The model under review builds one solid part; all positions refer to its coordinate system, in mm. Face numbers are marked on the shaded views. A direction names the side the tool comes from. Round coordinates to 2 decimals unless told otherwise and drop trailing zeros. Write each loop counter-clockwise with the first axis right and the second up, starting at its lowest first coordinate (ties: lowest second). Pieces come first, ordered by that corner, then holes. Notation, with made-up numbers: (69.5, 47) - (106.5, 47) arc R28 cw to (106.5, 72) - close; hole circle Ø7 at (89.25, 62.5). An arc over 180 degrees is marked (long way). Return JSON: item names as keys, results as strings.
from build123d import *

# Parameters (mm, degrees)
CYLINDER003_R     = 3
CYLINDER003_DEPTH = 10
PAD008_DEPTH      = 10
SKETCH032_R       = 1.625
POCKET023_DEPTH   = 55.910244
SKETCH033_W       = 20
SKETCH033_H       = 7
PAD009_DEPTH      = 7.5
SKETCH034_R       = 1.375
POCKET024_DEPTH   = 12
CHAMFER020_1_SIZE = 3.5
CHAMFER020_2_SIZE = 1
CHAMFER021_SIZE   = 0.5
CHAMFER022_SIZE   = 2


with BuildPart() as boardbracketscrewheadcylinder:
    # Cylinder003 → Cylinder003 (new body)
    with BuildSketch(Plane(origin=(0, 0.5, 24), x_dir=(1, 0, 0), z_dir=(0, 0, 1))):
        Circle(CYLINDER003_R)
    extrude(amount=CYLINDER003_DEPTH)


with BuildPart() as boardbracketpinschamfer022_final:
    # Sketch031 → Pad008 (new body, symmetric)
    with BuildSketch(Plane.YZ):
        Polygon((4.5, 21), (4.5, 24.911688), (-4.23971, 33.651398), (-7.975533, 34.909244), (-9.918525, 32.966252), (-9.211418, 32.259145), (-8.150758, 33.319805), (-5.32233, 31.905592), (-1.07969, 27.662951), (-25.828427, 2.914214), (-30.071068, 7.156854), (-31.485281, 9.985281), (-30.424621, 11.045942), (-31.131728, 11.753048), (-33.07472, 9.810056), (-31.714777, 5.972136), (-4.742641, -21), (4.5, -21), (4.5, -18), (-3.5, -18), (-23, 1.5), (-3.5, 21), align=None)
    extrude(amount=PAD008_DEPTH, both=True)

    # Sketch032 → Pocket023 (cut, through all)
    with BuildSketch(Plane.YX.offset(21)):
        with Locations((0.5, 0)):
            Circle(SKETCH032_R)
    extrude(amount=-POCKET023_DEPTH, mode=Mode.SUBTRACT)

    # Cut001: cut BoardBracketScrewHeadCylinder
    add(boardbracketscrewheadcylinder.part, mode=Mode.SUBTRACT)

    # Sketch033 → Pad009 (new body)
    with BuildSketch(Plane(origin=(0, -12.87132, -12.87132), x_dir=(1, 0, 0), z_dir=(0, -0.707107, -0.707107))):
        with Locations((0, 22.75)):
            Rectangle(SKETCH033_W, SKETCH033_H)
        with Locations((0, -7.5)):
            Rectangle(SKETCH033_W, SKETCH033_H)
    extrude(amount=PAD009_DEPTH)

    # Sketch034 → Pocket024 (cut)
    with BuildSketch(Plane(origin=(0, -18.174621, -18.174621), x_dir=(1, 0, 0), z_dir=(0, -0.707107, -0.707107))):
        with Locations((3.25, 22.75)):
            Circle(SKETCH034_R)
    pocket024 = extrude(amount=-POCKET024_DEPTH, mode=Mode.SUBTRACT)

    # Mirrored002: Pocket024 across Sketch034 V_Axis
    add(pocket024.mirror(Plane(origin=(0, -18.174621, -18.174621), x_dir=(0, -0.707107, -0.707107), z_dir=(1, 0, 0))), mode=Mode.SUBTRACT)

    # Chamfer020 1
    chamfer020_1_edges = [boardbracketpinschamfer022_final.edges().sort_by_distance(p)[0] for p in [
        (-10, -12.87132, -23.477922),
        (10, -12.87132, -23.477922),
    ]]
    chamfer(chamfer020_1_edges, length=CHAMFER020_1_SIZE)

    # Chamfer020 2
    chamfer020_2_edges = [boardbracketpinschamfer022_final.edges().sort_by_distance(p)[0] for p in [
        (-1.875, -34.2613, -2.087942),
        (1.875, -34.2613, -2.087942),
    ]]
    chamfer(chamfer020_2_edges, length=CHAMFER020_2_SIZE)

    # Chamfer021
    chamfer021_edges = [boardbracketpinschamfer022_final.edges().sort_by_distance(p)[0] for p in [
        (10, -4.917893, -20.824747),
        (10, -0.12132, -21),
        (10, 4.5, -19.5),
        (10, 0.5, -18),
        (10, -13.25, -8.25),
        (10, -13.25, 11.25),
        (10, 0.5, 21),
        (10, 4.5, 22.955844),
        (10, -30.778175, 8.571068),
        (10, -27.949747, 5.035534),
        (10, -13.454058, 15.288582),
        (10, -3.20101, 29.784271),
        (10, -6.736544, 32.612698),
    ]]
    chamfer(chamfer021_edges, length=CHAMFER021_SIZE)

    # Chamfer022
    chamfer022_edges = [boardbracketpinschamfer022_final.edges().sort_by_distance(p)[0] for p in [
        (8.25, -14.108757, -19.765611),
        (-8.25, -14.108757, -19.765611),
    ]]
    chamfer(chamfer022_edges, length=CHAMFER022_SIZE)


solid = boardbracketpinschamfer022_final.part
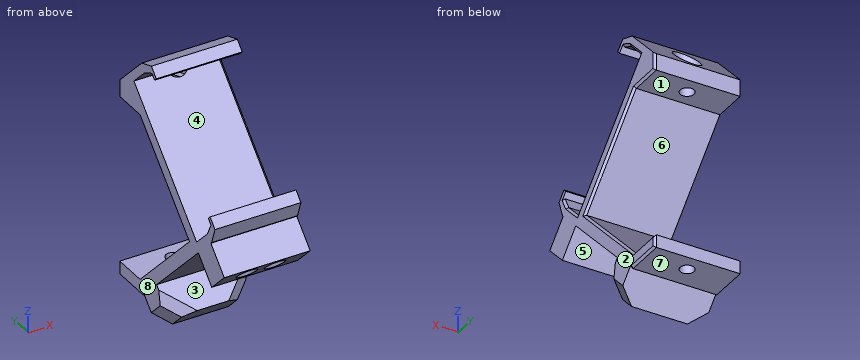
(1) Add section D-D (x = 0). Give the number of separate pieces and of enclosed holes in the cut face, plus the area to 3 significant figures.
Filled in:
{"separate pieces": "4", "enclosed holes": "0", "area": "355 mm2"}
(2) For the marked faces 1, 2, 3, 4 and 5, list the 3-axis set-ups (+Z, -Z, +X, -X, +Y, -Y) from which the entire face can be reached by the end or side of a thin tool; tool diameter is ignored.
Filled in:
{"face 1": "+X, -X, +Y", "face 2": "+Z, -Z, +X, +Y, -Y", "face 3": "+X, -X, -Y", "face 4": "+X, -X", "face 5": "-Z, +X, -X"}
(3) Add section A-A (y = -18). Write out the cut boundary in (x, z).
Filled in:
{"outline": "(-10, -7.74) - (10, -7.74) - (10, -4.21) - (9.5, -3.5) - (-10, -3.5) - close; (-10, 6.5) - (9.5, 6.5) - (10, 7.21) - (10, 10.04) - (9.5, 10.74) - (-10, 10.74) - close"}
(4) Clearance check with flat-ended pins moving along their axes: pin 1 Ø1.5 at (x, z) = (7, -15) entering from +Y; pin 2 Ø4 at (x, y) = (0, 0.5) entering from +Z; pin 3 Ø8 at (x, y) = (0, 0.5) entering from -Z. State where each tip first meets the part, or that it passes through.
Filled in:
{"pin 1": "stops at y = -5.75", "pin 2": "stops at z = 24", "pin 3": "stops at z = -21"}
(5) Mouldability with a two-part tool opening along Z and no side actions: class the marked faces 6, 7 and 8 as released by +Z, released by -Z, zero draft, split by the parting line, or undercut.
Filled in:
{"face 6": "undercut", "face 7": "released by -Z", "face 8": "zero draft"}
(6) Add section C-C (z = 19). Write out the cut boundary in (x, y), plus the area to 3 significant figures.
Filled in:
{"outline": "(-10, -9.74) - (9.5, -9.74) - (10, -9.04) - (10, -6.21) - (9.5, -5.5) - (-10, -5.5) - close", "area": "84.5 mm2"}
(7) Wall thickness on line 1 (Z direction, x = 8.75, y = -10.5); line 2 (Z direction, x = 9, y = -9); line 3 (X direction, y = 0, z = 22): over which ranges is each line inside the solid? List them lowest first.
Filled in:
{"line 1": "z = -22.67 to -16.16, -15.24 to -11, 14 to 18.24", "line 2": "z = -23.81 to -12.5, 15.5 to 19.74, 32.47 to 33.88", "line 3": "x = -10 to -1.55, 1.55 to 10"}
(8) Add section B-B (y = 0.5). Write out the cut boundary in (x, z) (3 decimals), plus the area to 3 significant figures.
Filled in:
{"outline": "(-10, -21) - (-1.625, -21) - (-1.625, -18) - (-10, -18) - close; (-10, 21) - (-1.625, 21) - (-1.625, 24) - (-3, 24) - (-3, 28.912) - (-10, 28.912) - close; (1.625, -21) - (9.5, -21) - (10, -20.5) - (10, -18.5) - (9.5, -18) - (1.625, -18) - close; (1.625, 21) - (9.5, 21) - (10, 21.5) - (10, 28.912) - (3, 28.912) - (3, 24) - (1.625, 24) - close", "area": "169 mm2"}
